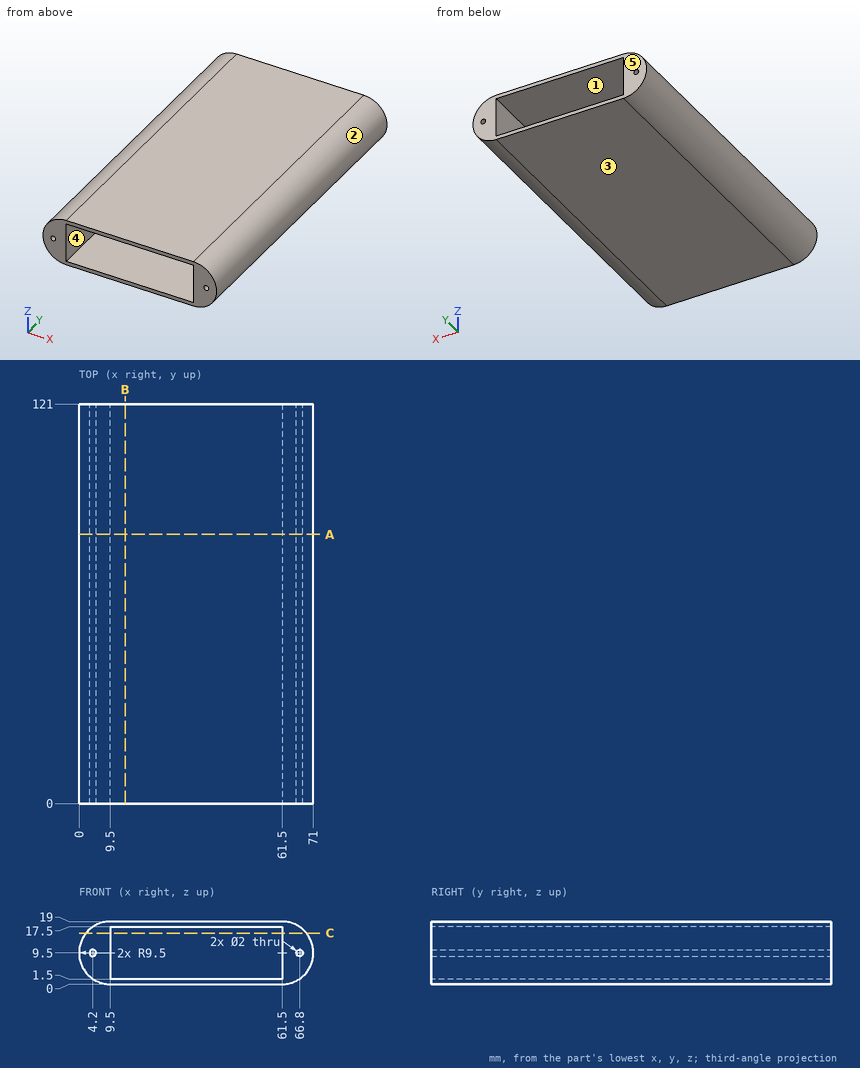
Design review of the part shown in the three views and the two pictorial views. Dimensions are in mm from the part's minimum x, y and z. A direction names the side the tool comes from. Round coordinates to 2 decimals unless told otherwise and drop trailing zeros. Order: outer loops, then holes, each group sorted by start corner. A loop starts at its lowest first (then second) coordinate and runs counter-clockwise, first axis right, second up. Notation, with made-up numbers: (86.5, -18) - (98.5, -18) arc R5 ccw to (98.5, -13) - close; hole circle Ø2 at (68, 34). An arc over 180 degrees is marked (long way). Answer in a Markdown table with one row per item.
(1) Take a section at B-B on x = 14. Write out the cut boundary in (y, z), plus the area to 3 significant figures.
Result set:
| item | result |
|---|---|
| outline | (0, 0) - (121, 0) - (121, 1.5) - (0, 1.5) - close; (0, 17.5) - (121, 17.5) - (121, 19) - (0, 19) - close |
| area | 363 mm2 |
(2) Take a section at C-C on z = 15.5. Write out the cut boundary in (x, y), plus the area to 3 significant figures.
Result set:
| item | result |
|---|---|
| outline | (2.13, 0) - (9.5, 0) - (9.5, 121) - (2.13, 121) - close; (61.5, 0) - (68.87, 0) - (68.87, 121) - (61.5, 121) - close |
| area | 1,780 mm2 |
(3) Clearance check with flat-ended pins moving along their axes: P1, Ø4, axis at x = 43, z = 5, coming from the +Y side; P2, Ø2, axis at y = 51, z = 4, coming from the -X side. State where each tip first meets the part, or that it passes through.
Result set:
| item | result |
|---|---|
| P1 | passes through |
| P2 | stops at x = 1.13 |
(4) Machinability: for the marked faces 1 and 2, which of the approach directions +Z, -Z, +X, -X, +Y, -Y give a long, thin tool a straight path to every point of the face, cutting with its end or side? Answer none if there is none.
Result set:
| item | result |
|---|---|
| face 1 | +Y, -Y |
| face 2 | +X, +Y, -Y |
(5) Mouldability with a two-part tool opening along Z and no side actions: class the marked faces 3, 4 and 5 as released by +Z, released by -Z, zero draft, split by the parting line, or undercut.
Result set:
| item | result |
|---|---|
| face 3 | released by -Z |
| face 4 | undercut |
| face 5 | zero draft |
(6) Take a section at A-A on y = 81.5. Write out the cut boundary in (x, z), plus the area to 3 significant figures.
Result set:
| item | result |
|---|---|
| outline | (9.5, 0) - (61.5, 0) arc R9.5 ccw to (61.5, 19) - (9.5, 19) arc R9.5 ccw to start; hole circle Ø2 at (4.2, 9.5); hole (9.5, 1.5) - (61.5, 1.5) - (61.5, 17.5) - (9.5, 17.5) - close; hole circle Ø2 at (66.8, 9.5) |
| area | 433 mm2 |
(7) For line 1 (Z direction, x = 15, y = 13.5); line 2 (X direction, y = 9, z = 8.75); line 3 (X direction, y = 97, z = 6), list the stretches that pass through material, from the lowest coordinate up. Write a range as from..to.
Result set:
| item | result |
|---|---|
| line 1 | z = 0..1.5, 17.5..19 |
| line 2 | x = 0.03..3.54, 4.86..9.5, 61.5..66.14, 67.46..70.97 |
| line 3 | x = 0.67..9.5, 61.5..70.33 |
